```python
from build123d import *

# Parameters (mm, degrees)
SKETCH1_R                = 2.75
BOSS_EXTRUDE1_DEPTH      = 2
SKETCH2_W                = 3
SKETCH2_H                = 100
BOSS_EXTRUDE2_DEPTH      = 2
SKETCH3_W                = 60
SKETCH3_H                = 3
BOSS_EXTRUDE3_DEPTH      = 2
CHAMFER1_SIZE            = 2
CHAMFER1_OF_MIRROR1_SIZE = 2
SKETCH5_W                = 35
SKETCH5_H                = 30
BOSS_EXTRUDE4_DEPTH      = 2
CHAMFER2_SIZE            = 3
CUT_EXTRUDE1_DEPTH       = 122.80201158
CUT_EXTRUDE1_DEPTH_BACK  = 122.80201158
CUT_EXTRUDE2_DEPTH       = 116.086836888
CUT_EXTRUDE2_DEPTH_BACK  = 116.086836888
SKETCH7_R                = 2.6
BOSS_EXTRUDE5_DEPTH      = 35
CUT_EXTRUDE3_DEPTH       = 116.086836888
CUT_EXTRUDE3_DEPTH_BACK  = 116.086836888
SKETCH9_W                = 3
SKETCH9_H                = 2


# Some blends are built 0.0001 mm under size
with BuildPart() as part:
    # Sketch1 → Boss-Extrude1 (new body)
    with BuildSketch(Plane(origin=(0, 0, 0), x_dir=(1, 0, 0), z_dir=(0, 1, 0))):
        Polygon((-17.5, 42.995), (-17.5, -42.995), (-36.7, -42.995), (-36.7, -109.005), (36.7, -109.005), (36.7, -42.995), (17.5, -42.995), (17.5, 42.995), (36.7, 42.995), (36.7, 109.005), (-36.7, 109.005), (-36.7, 42.995), align=None)
        with Locations(Location((-31.7, 102.855, 0), (0, 0, 270))):
            Circle(SKETCH1_R, mode=Mode.SUBTRACT)
        with Locations(Location((-31.7, 49.145, 0), (0, 0, 270))):
            Circle(SKETCH1_R, mode=Mode.SUBTRACT)
        with Locations(Location((31.7, 49.145, 0), (0, 0, 270))):
            Circle(SKETCH1_R, mode=Mode.SUBTRACT)
        with Locations(Location((31.7, 102.855, 0), (0, 0, 270))):
            Circle(SKETCH1_R, mode=Mode.SUBTRACT)
        with Locations(Location((31.7, -102.855, 0), (0, 0, 270))):
            Circle(SKETCH1_R, mode=Mode.SUBTRACT)
        with Locations(Location((31.7, -49.145, 0), (0, 0, 270))):
            Circle(SKETCH1_R, mode=Mode.SUBTRACT)
        with Locations(Location((-31.7, -49.145, 0), (0, 0, 270))):
            Circle(SKETCH1_R, mode=Mode.SUBTRACT)
        with Locations(Location((-31.7, -102.855, 0), (0, 0, 270))):
            Circle(SKETCH1_R, mode=Mode.SUBTRACT)
    extrude(amount=BOSS_EXTRUDE1_DEPTH)

    # Sketch2 → Boss-Extrude2 (add)
    with BuildSketch(Plane(origin=(0, 2, 0), x_dir=(1, 0, 0), z_dir=(0, 1, 0))):
        with Locations((12, -50)):
            Rectangle(SKETCH2_W, SKETCH2_H)
        with Locations((0, -50)):
            Rectangle(SKETCH2_W, SKETCH2_H)
        with Locations((-12, -50)):
            Rectangle(SKETCH2_W, SKETCH2_H)
    boss_extrude2 = extrude(amount=BOSS_EXTRUDE2_DEPTH)

    # Sketch3 → Boss-Extrude3 (add)
    with BuildSketch(Plane(origin=(0, 2, 0), x_dir=(1, 0, 0), z_dir=(0, 1, 0))):
        with Locations((0, -91)):
            Rectangle(SKETCH3_W, SKETCH3_H)
        with Locations((0, -61)):
            Rectangle(SKETCH3_W, SKETCH3_H)
        with Locations((0, -76)):
            Rectangle(SKETCH3_W, SKETCH3_H)
    boss_extrude3 = extrude(amount=BOSS_EXTRUDE3_DEPTH)

    # Chamfer1
    chamfer1_edges = [part.edges().sort_by_distance(p)[0] for p in [
        (30, 4, 61),
        (30, 4, 76),
        (30, 4, 91),
        (12, 4, 100),
        (0, 4, 100),
        (-12, 4, 100),
        (-30, 4, 91),
        (-30, 4, 76),
        (-30, 4, 61),
    ]]
    chamfer(chamfer1_edges, length=CHAMFER1_SIZE - 0.0001)  # a hair under: the kernel refuses the full size

    # Mirror1: Boss-Extrude2, Boss-Extrude3 across plane
    add(boss_extrude2.mirror(Plane.XY))
    add(boss_extrude3.mirror(Plane.XY))

    # Chamfer1 of Mirror1
    chamfer1_of_mirror1_edges = [part.edges().sort_by_distance(p)[0] for p in [
        (30, 4, -61),
        (30, 4, -76),
        (30, 4, -91),
        (12, 4, -100),
        (0, 4, -100),
        (-12, 4, -100),
        (-30, 4, -91),
        (-30, 4, -76),
        (-30, 4, -61),
    ]]
    chamfer(chamfer1_of_mirror1_edges, length=CHAMFER1_OF_MIRROR1_SIZE - 0.0001)  # a hair under: the kernel refuses the full size

    # Sketch5 → Boss-Extrude4 (add)
    with BuildSketch(Plane(origin=(0, 4, 0), x_dir=(1, 0, 0), z_dir=(0, 1, 0))):
        Rectangle(SKETCH5_W, SKETCH5_H)
    extrude(amount=-BOSS_EXTRUDE4_DEPTH)

    # Chamfer2
    # the kernel refuses this chamfer: 3 mm, written as the material it adds along each edge
    with BuildSketch(Plane(origin=(17.5, 2, 15), x_dir=(0, 0.9996219169112969, -0.027495876610586202), z_dir=(-1, 0, 0))) as chamfer2_piece_1_section:
        Polygon((CHAMFER2_SIZE * 0.999621916911, -CHAMFER2_SIZE * 0.0274958766106), (-CHAMFER2_SIZE * 0.0274958766106, -CHAMFER2_SIZE * 0.999621916911), (0, 0), align=None)
    chamfer2_piece_1 = extrude(amount=11.715048964, mode=Mode.PRIVATE)
    chamfer2_piece_1 = split(chamfer2_piece_1, bisect_by=Plane(origin=(15.5, 4, 16.092091005), z_dir=(0, -1, 0)), keep=Keep.TOP, mode=Mode.PRIVATE)
    add(chamfer2_piece_1)
    with BuildSketch(Plane(origin=(18.215048964, 2, 15), x_dir=(0, 0.9996219169112969, -0.027495876610586202), z_dir=(-1, 0, 0))) as chamfer2_piece_2_section:
        Polygon((CHAMFER2_SIZE * 0.999621916911, -CHAMFER2_SIZE * 0.0274958766106), (-CHAMFER2_SIZE * 0.0274958766106, -CHAMFER2_SIZE * 0.999621916911), (0, 0), align=None)
    chamfer2_piece_2 = extrude(amount=24.430097928, mode=Mode.PRIVATE)
    chamfer2_piece_2 = split(chamfer2_piece_2, bisect_by=Plane(origin=(14, 4, 16.092091005), z_dir=(0, -1, 0)), keep=Keep.TOP, mode=Mode.PRIVATE)
    chamfer2_piece_2 = split(chamfer2_piece_2, bisect_by=Plane(origin=(17.5, 2.79312586, 16.092091005), z_dir=(-1, 0, 0)), keep=Keep.TOP, mode=Mode.PRIVATE)
    add(chamfer2_piece_2)
    with BuildSketch(Plane(origin=(6.215048964, 2, 15), x_dir=(0, 0.9996219169112969, -0.027495876610586202), z_dir=(-1, 0, 0))) as chamfer2_piece_3_section:
        Polygon((CHAMFER2_SIZE * 0.999621916911, -CHAMFER2_SIZE * 0.0274958766106), (-CHAMFER2_SIZE * 0.0274958766106, -CHAMFER2_SIZE * 0.999621916911), (0, 0), align=None)
    chamfer2_piece_3 = extrude(amount=24.430097928, mode=Mode.PRIVATE)
    chamfer2_piece_3 = split(chamfer2_piece_3, bisect_by=Plane(origin=(2.357524482, 4, 16.092091005), z_dir=(0, -1, 0)), keep=Keep.TOP, mode=Mode.PRIVATE)
    chamfer2_piece_3 = split(chamfer2_piece_3, bisect_by=Plane(origin=(-17.5, 2.79312586, 16.092091005), z_dir=(1, 0, 0)), keep=Keep.TOP, mode=Mode.PRIVATE)
    add(chamfer2_piece_3)
    with BuildSketch(Plane(origin=(-5.784951036, 2, 15), x_dir=(0, 0.9996219169112969, -0.027495876610586202), z_dir=(-1, 0, 0))) as chamfer2_piece_4_section:
        Polygon((CHAMFER2_SIZE * 0.999621916911, -CHAMFER2_SIZE * 0.0274958766106), (-CHAMFER2_SIZE * 0.0274958766106, -CHAMFER2_SIZE * 0.999621916911), (0, 0), align=None)
    chamfer2_piece_4 = extrude(amount=11.715048964, mode=Mode.PRIVATE)
    chamfer2_piece_4 = split(chamfer2_piece_4, bisect_by=Plane(origin=(-9.642475518, 4, 16.092091005), z_dir=(0, -1, 0)), keep=Keep.TOP, mode=Mode.PRIVATE)
    add(chamfer2_piece_4)

    # Sketch6 → Cut-Extrude1 (cut, two sides: drawn at the far end of the back side and taken through both)
    with BuildSketch(Plane(origin=(17.5, 0, 0), x_dir=(0, 0, -1), z_dir=(1, 0, 0)).offset(-CUT_EXTRUDE1_DEPTH_BACK)):
        Polygon((-13, 0), (-13, 2), (15, 2), (15, 4), (109.005, 4), (109.005, 0), align=None)
    extrude(amount=CUT_EXTRUDE1_DEPTH + CUT_EXTRUDE1_DEPTH_BACK, mode=Mode.SUBTRACT)

    # Sketch7 → Cut-Extrude2 (cut, two sides: drawn at the far end of the back side and taken through both)
    with BuildSketch(Plane(origin=(0, 4, 0), x_dir=(1, 0, 0), z_dir=(0, 1, 0)).offset(-CUT_EXTRUDE2_DEPTH_BACK)):
        with Locations(Location((-10, -8, 0), (0, 0, 270))):
            Circle(SKETCH7_R)
        with Locations(Location((-10, 8, 0), (0, 0, 270))):
            Circle(SKETCH7_R)
        with Locations(Location((10, 8, 0), (0, 0, 270))):
            Circle(SKETCH7_R)
        with Locations(Location((10, -8, 0), (0, 0, 270))):
            Circle(SKETCH7_R)
    extrude(amount=CUT_EXTRUDE2_DEPTH + CUT_EXTRUDE2_DEPTH_BACK, mode=Mode.SUBTRACT)

    # Sketch8 → Boss-Extrude5 (add)
    with BuildSketch(Plane(origin=(17.5, 0, 0), x_dir=(0, 0, -1), z_dir=(1, 0, 0))):
        Polygon((15, 4), (17, 2), (15, 2), align=None)
    extrude(amount=-BOSS_EXTRUDE5_DEPTH)

    # Sketch9 → Cut-Extrude3 (cut, two sides: drawn at the far end of the back side and taken through both)
    with BuildSketch(Plane(origin=(0, 4, 0), x_dir=(1, 0, 0), z_dir=(0, 1, 0)).offset(-CUT_EXTRUDE3_DEPTH_BACK)):
        with Locations((-12, 16)):
            Rectangle(SKETCH9_W, SKETCH9_H)
        with Locations((0, 16)):
            Rectangle(SKETCH9_W, SKETCH9_H)
        with Locations((12, 16)):
            Rectangle(SKETCH9_W, SKETCH9_H)
    extrude(amount=CUT_EXTRUDE3_DEPTH + CUT_EXTRUDE3_DEPTH_BACK, mode=Mode.SUBTRACT)


solid = part.part
```
For this review, take the finished solid that the model builds, in its own axes (mm). A direction names the side the tool comes from. Coordinates: 2 decimals unless noted, no trailing zeros. Loops run counter-clockwise (first coordinate to the right, second up) from the corner with the lowest first, then second, coordinate; pieces in that order, holes last.
1. For faces 1 (the cylindrical face through (7.46, 2.99, -8.56)), 2 (the flat face through (6, 2, 38)), list the 3-axis set-ups (+Z, -Z, +X, -X, +Y, -Y) from which the entire face can be reached by the end or side of a thin tool; tool diameter is ignored.
2. Mouldability with a two-part tool opening along X and no side actions: class faces 3 (the flat face through (-17.5, 2.5, 12.6)), 4 (the flat face through (6, 2, 83)), 5 (the flat face through (0, 4, 42)) as +X half, -X half, draft (parallel to the pull), parting line (faces both ways), or undercut.
3. Add section A-A, the plane x = -31.7. Give the boundary of the cut face in (y, z) (3 decimals), then the cut area to 3 significant figures.
4. Add section D-D, the plane z = 24. Give the boundary of the cut face in (x, y), then the cut area to 3 significant figures.
5. Insertion check: P1, Ø1, axis at y = 3.5, z = 71, coming from the +X side; P2, Ø3, axis at x = 4.5, z = 20.5, coming from the +Y side; P3, Ø0.6, axis at y = 2.5, z = -15.5, coming from the +X side. Each pin has a flat end and moves straight along its axis. Give the tip position at first contact, or say it passes through.
6. For line 1 (X direction, y = 2.55, z = 52); line 2 (Z direction, x = 10, y = 2.7); line 3 (X direction, y = 3.05, z = 8), list the stretches that pass through material, from the lowest coordinate up.
7. Add section C-C, the plane x = -6. Give the boundary of the cut face in (y, z) (3 decimals).
8. Add section B-B, the plane z = 8. Give the boundary of the cut face in (x, y).
Result:
1. face 1: +Y, -Y
1. face 2: +Y
2. face 3: -X half
2. face 4: undercut
2. face 5: draft
3. outline: (0, 42.995) - (2, 42.995) - (2, 46.395) - (0, 46.395) - close; (0, 51.895) - (2, 51.895) - (2, 100.105) - (0, 100.105) - close; (0, 105.605) - (2, 105.605) - (2, 109.005) - (0, 109.005) - close
3. area: 110 mm2
4. outline: (-17.5, 0) - (17.5, 0) - (17.5, 2) - (13.5, 2) - (13.5, 4) - (10.5, 4) - (10.5, 2) - (1.5, 2) - (1.5, 4) - (-1.5, 4) - (-1.5, 2) - (-10.5, 2) - (-10.5, 4) - (-13.5, 4) - (-13.5, 2) - (-17.5, 2) - close
4. area: 88.0 mm2
5. P1: stops at x = 13.5
5. P2: stops at y = 2
5. P3: stops at x = 17.5
6. line 1: x = -13.5 to -10.5, -1.5 to 1.5, 10.5 to 13.5
6. line 2: z = -16.3 to -10.6, -5.4 to 5.4, 10.6 to 17.3, 59.5 to 62.5, 74.5 to 77.5, 89.5 to 92.5
6. line 3: x = -17.5 to -12.6, -7.4 to 7.4, 12.6 to 17.5
7. outline: (0, 13) - (2, 13) - (2, -17) - (4, -15) - (4, 16) - (2, 18) - (2, 59.5) - (4, 59.5) - (4, 62.5) - (2, 62.5) - (2, 74.5) - (4, 74.5) - (4, 77.5) - (2, 77.5) - (2, 89.5) - (4, 89.5) - (4, 92.5) - (2, 92.5) - (2, 109.005) - (0, 109.005) - close
8. outline: (-17.5, 2) - (-12.6, 2) - (-12.6, 4) - (-17.5, 4) - close; (-7.4, 2) - (7.4, 2) - (7.4, 4) - (-7.4, 4) - close; (12.6, 2) - (17.5, 2) - (17.5, 4) - (12.6, 4) - close
